Work out the finished part from the listing and answer in its coordinate system (mm). A direction names the side the tool comes from. Coordinates: 2 decimals unless noted, no trailing zeros. Write each loop counter-clockwise with the first axis right and the second up, starting at its lowest first coordinate (ties: lowest second). Pieces come first, ordered by that corner, then holes. Notation, with made-up numbers: (78.5, -29.75) - (110.5, -29.75) arc R12 cw to (110.5, -6.75) - close; hole circle Ø8 at (47.25, -15.75). An arc over 180 degrees is marked (long way). One line per item, written item: value.
```python
from build123d import *

# Parameters (mm, degrees)
F0_W          = 100
F0_H          = 100
F1_DEPTH      = 100
F2_R          = 35
F3_DEPTH      = 170
F4_R          = 35
F5_DEPTH      = 161.955625
F5_DEPTH_BACK = 76.630928
F6_R          = 35
F7_DEPTH      = 1320.8


with BuildPart() as f1:
    # F0 (on Front) → F1 (new body)
    with BuildSketch(Plane.XZ):
        Rectangle(F0_W, F0_H)
    extrude(amount=F1_DEPTH)

    # F2 (on Front) → F3 (join)
    with BuildSketch(Plane.XZ):
        Circle(F2_R)
    extrude(amount=F3_DEPTH)

    # F4 (on Front) → F5 (join, two sides)
    with BuildSketch(Plane.XZ) as f5_sk:
        Circle(F4_R)
    extrude(amount=F5_DEPTH)
    extrude(f5_sk.sketch, amount=-F5_DEPTH_BACK)

    # F6 (on Right) → F7 (cut)
    with BuildSketch(Plane.YZ):
        with Locations((-34.9987, 0.301605)):
            Circle(F6_R)
    extrude(amount=-F7_DEPTH, mode=Mode.SUBTRACT)


solid = f1.part
```
Item 1: Section A-A, the plane y = -35 is taken. Determine the outline of the cut face in (x, z).
Evaluation:
outline: (-50, -50) - (50, -50) - (50, 50) - (-50, 50) - (-50, 35.3) - (0, 35.3) - (0, -34.7) - (-50, -34.7) - close
Item 2: Given pin 1 (6 mm diameter, centred on x = 7.5, y = 18.5, fed in from +Z); pin 2 (21 mm diameter, centred on y = -48, z = -10, fed in from -X); pin 3 (6 mm diameter, centred on y = 13, z = -14.5, fed in from +X), each flat-ended and moving along its own axis, determine where each tip first touches the part or whether it passes through.
Evaluation:
pin 1: stops at z = 34.71
pin 2: stops at x = 0
pin 3: stops at x = 33.06
Item 3: Section B-B, the plane x = 16 is taken. Determine the outline of the cut face in (y, z).
Evaluation:
outline: (-170, -31.13) - (-100, -31.13) - (-100, -50) - (0, -50) - (0, -31.13) - (76.63, -31.13) - (76.63, 31.13) - (0, 31.13) - (0, 50) - (-100, 50) - (-100, 31.13) - (-170, 31.13) - close
Item 4: Section C-C, the plane z = -44 is taken. Determine the outline of the cut face in (x, y).
Evaluation:
outline: (-50, -100) - (50, -100) - (50, 0) - (-50, 0) - close
Item 5: Determine the mould class of faces 1 (the face through (-24.65, -69.965, 1.84)), 2 (the face through (0, 76.631, 0)), 3 (the face through (-28, -135, -21)) for opening direction Z: +Z half, -Z half, draft (parallel to the pull), parting line (faces both ways), or undercut.
Evaluation:
face 1: undercut
face 2: draft
face 3: parting line
Item 6: Which of the six approach directions +Z, -Z, +X, -X, +Y, -Y give full straight-line access (tool end or side, diameter ignored) to faces 4 (the face through (0, -170, 0)), 5 (the face through (-34, -100, 12)), 6 (the face through (-34, 0, 12)), 7 (the face through (-50, -72, -1)), 8 (the face through (0, -35, 1))?
Evaluation:
face 4: +Z, -Z, +X, -X, -Y
face 5: -Y
face 6: +Y
face 7: +Z, -Z, -X, +Y, -Y
face 8: -X
Item 7: Consider probe 1 along Y at (x, z) = (37, -42); probe 2 along X at (y, z) = (-26.5, 24); probe 3 along Y at (x, z) = (-41, 21). Determine where each line is inside the solid, lowest interval first.
Evaluation:
probe 1: y = -100 to 0
probe 2: x = 0 to 50
probe 3: y = -100 to -63.22, -6.78 to 0
Item 8: Section D-D, the plane x = -27 is taken. Determine the outline of the cut face in (y, z), then the cut area to 3 significant figures.
Evaluation:
outline: (-170, -22.27) - (-100, -22.27) - (-100, -50) - (0, -50) - (0, -22.27) - (76.63, -22.27) - (76.63, 22.27) - (0, 22.27) - (0, 50) - (-100, 50) - (-100, 22.27) - (-170, 22.27) - close; hole circle Ø70 at (-35, 0.3)
area: 12,700 mm2
